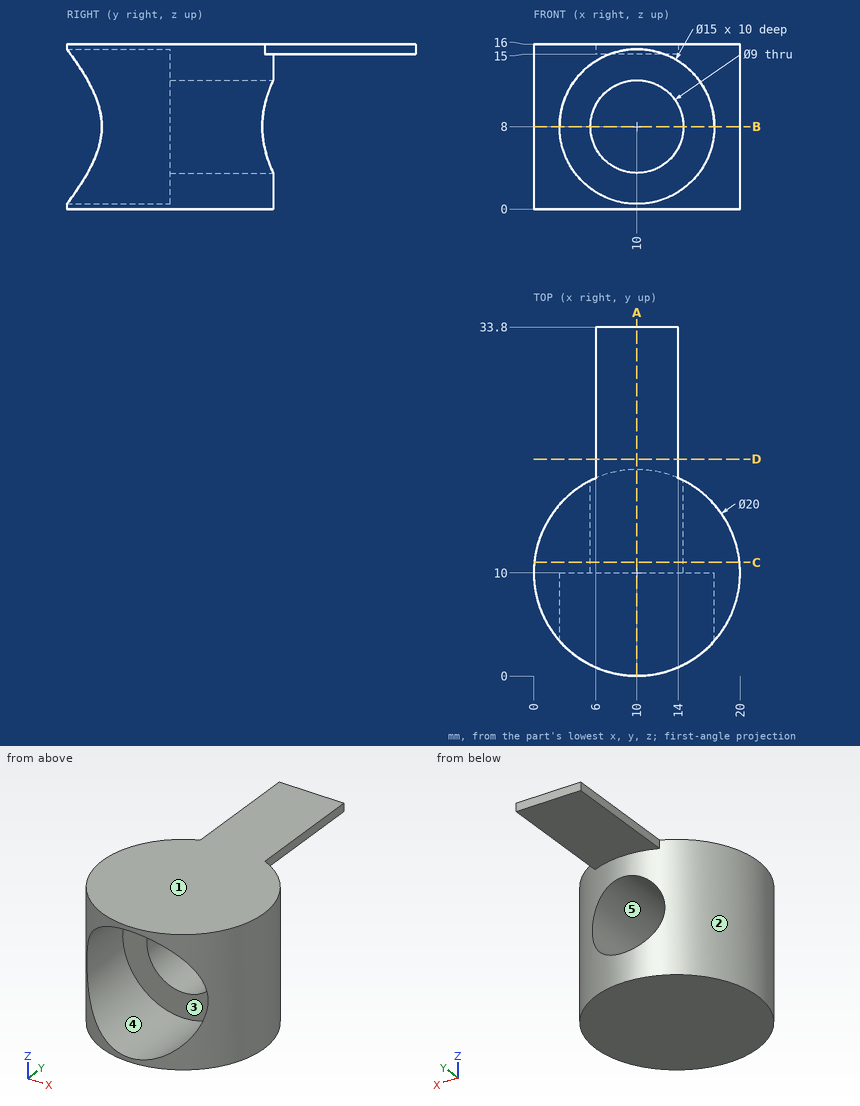
For this review, use the dimensioned drawing (mm, ordinates from the lowest corner) and the shaded views. A direction names the side the tool comes from. Give positions to 0.01 mm unless a question says otherwise; leave off trailing zeros. Order: outer loops, then holes, each group sorted by start corner. A loop starts at its lowest first (then second) coordinate and runs counter-clockwise, first axis right, second up.
1) Insertion check: pin 1 (1.5 mm diameter, centred on y = 21.5, z = 3, fed in from -X); pin 2 (7.5 mm diameter, centred on x = 8.5, z = 5, fed in from -Y); pin 3 (4 mm diameter, centred on x = 9, y = 30, fed in from -Z); pin 4 (1.1 mm diameter, centred on y = 27, z = 15.5, fed in from +X). Each pin has a flat end and moves straight along its axis. Give the tip position at first contact, or say it passes through.
2) The part is to be moulded in two halves that separate along X. For the marked faces 1, 2 and 3, say which applies: released by +X, released by -X, zero draft, split by the parting line, or undercut.
3) Wall thickness on line 1 (Z direction, x = 10.25, y = 14); line 2 (Z direction, x = 13.75, y = 3); line 3 (X direction, y = 4.5, z = 7.25): over which ranges is each line inside the solid? List them lowest first.
4) Take a section at D-D (y = 21). Give the boundary of the cut face in (x, z).
5) For the marked faces 4 and 5, list the 3-axis set-ups (+Z, -Z, +X, -X, +Y, -Y) from which the entire face can be reached by the end or side of a thin tool; tool diameter is ignored.
6) Take a section at A-A (x = 10). Give the boundary of the cut face in (y, z).
7) Take a section at C-C (y = 11). Give the boundary of the cut face in (x, z), then the cut area to 3 significant figures.
8) Take a section at B-B (z = 8). Give the boundary of the cut face in (x, y).
Derived:
1. pin 1: passes through
1. pin 2: stops at y = 10
1. pin 3: stops at z = 15
1. pin 4: stops at x = 14
2. face 1: zero draft
2. face 2: split by the parting line
2. face 3: undercut
3. line 1: z = 0 to 3.51, 12.49 to 16
3. line 2: z = 0 to 1.5, 14.5 to 16
3. line 3: x = 1.65 to 2.54, 17.46 to 18.35
4. outline: (6, 15) - (14, 15) - (14, 16) - (6, 16) - close
5. face 4: -Y
5. face 5: +Y, -Y
6. outline: (0, 0) - (20, 0) - (20, 3.5) - (10, 3.5) - (10, 0.5) - (0, 0.5) - close; (0, 15.5) - (10, 15.5) - (10, 12.5) - (20, 12.5) - (20, 15) - (33.8, 15) - (33.8, 16) - (0, 16) - close
7. outline: (0.05, 0) - (19.95, 0) - (19.95, 16) - (0.05, 16) - close; hole circle Ø9 at (10, 8)
7. area: 255 mm2
8. outline: (2.5, 3.39) - (2.5, 10) - (5.5, 10) - (5.5, 18.93) arc R10 ccw to start; (14.5, 10) - (17.5, 10) - (17.5, 3.39) arc R10 ccw to (14.5, 18.93) - close
